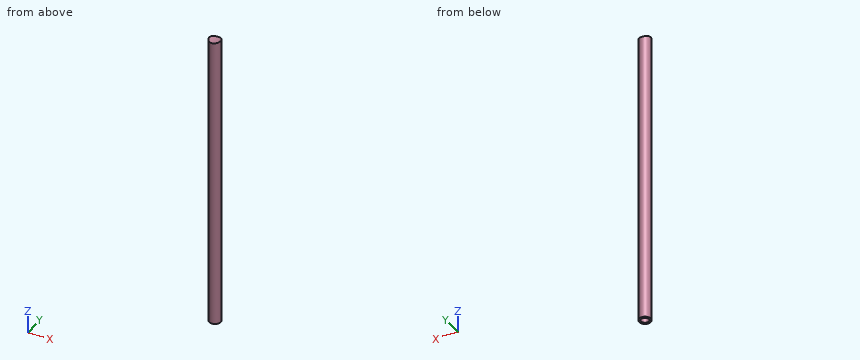
Autodesk Inventor part; units mm, degrees
ref_plane "Start Plane" through (0, 0, 0) normal (0, 0, 1) x (1, 0, 0)
ref_plane "End Plane" through (0, 0, 340) normal (0, 0, 1) x (1, 0, 0)
ref_plane "YZ Plane" through (0, 0, 0) normal (1, 0, 0) x (0, 1, 0)
ref_plane "Start Plane" through (0, 0, 0) normal (0, 0, 1) x (1, 0, 0)
ref_plane "End Plane" through (0, 0, 340) normal (0, 0, 1) x (1, 0, 0)
sketch "Sketch" plane through (0, 0, 0) normal (0, 0, 1) x (1, 0, 0)
  circle A0 centre (0, 0) radius 6.35
  dimension "d0" = 12.7
extrude "Body" add sketch "Sketch" along normal up to surface (340 mm away) from surface at 0
sketch "Sketch2" plane through (0, 0, 0) normal (0, 0, 1) x (1, 0, 0)
  line L0 (0, 0) -> (10, 0)
ref_plane "Work Plane3" through (0, 0, 0) normal (0, -1, 0) x (1, 0, 0)
sketch "Sketch4" plane through (0, 0, 0) normal (0, 1, 0) x (-1, 0, 0)
  line L0 (-6.35, 340) -> (6.35, 340)
  circle A0 centre (0, 340) radius 20
  point P0 (0, 0)
  dimension "d11" = 40
extrude "Extrusion2" cut sketch "Sketch4" along normal through all both and the other way through all
sketch "Sketch5" plane through (0, 0, 0) normal (0, 0, -1) x (-1, 0, 0)
  circle A0 centre (0, 0) radius 4.2164
  dimension "d12" = 8.4328
extrude "Extrusion3" cut sketch "Sketch5" against normal blind 50.8
thread "Thread1"
sketch "Sketch3" plane through (0, 0, 0) normal (0, -1, 0) x (1, 0, 0)
  line L0 (-2, 0) -> (12, 0)
  line L1 (-2, 340) -> (12, 340)
  dimension "d7" = 340
equation "\"d0\" = Diam"
equation "\"d1\" = G_L"
equation "\"Diam\" = 12.7"
equation "\"G_L\" = d7"
equation "\"G_OFFSET_START\" = 0"
equation "\"G_OFFSET_END\" = 0"
equation "\"d5\" = G_OFFSET_END + B_L"
equation "\"B_L\" = 340"
properties part number "ANSI/AISC Rolled Steel - 1/2-13.386, RB" material "Steel, Mild"
Verification items for the finished model (mm, model axes). Coordinates: 2 decimals unless noted, no trailing zeros. Write each loop counter-clockwise with the first axis right and the second up, starting at its lowest first coordinate (ties: lowest second). Pieces come first, ordered by that corner, then holes. Notation, with made-up numbers: (-37, 45) - (-26, 45) arc R8 ccw to (-26, 59) - close; hole circle Ø11 at (68.25, 27.5). An arc over 180 degrees is marked (long way). One line per question, with ' | ' between items. Start each with the question number.
1. Section check B-B (x = 0). Enter the section's corners in (y, z), plus the area to 3 significant figures.
2. Gauge pin test, flat ends, axial feed: P1, Ø1, axis at x = -0.5, y = -4.5, coming from the +Z side (3 decimals); P2, Ø3, axis at x = 3.5, z = 254, coming from the +Y side; P3, Ø4, axis at x = 0, y = -5, coming from the -Z side; P4, Ø1.5, axis at x = -3.5, z = 244, coming from the -Y side. Record the tip position at first contact, or that the pin passes through.
3. Material ranges on line 1 along Y through (x, z) = (0, 20.5); line 2 along Z through (x, y) = (-0.25, 3.5); line 3 along X through (y, z) = (-0.25, 288), recorded low to high.
4. Section check C-C (z = 88). Enter the section's corners in (x, y).
5. Section check A-A (y = 0). Enter the section's corners in (x, z).
Computed values:
1) outline: (-6.35, 0) - (-4.22, 0) - (-4.22, 50.8) - (4.22, 50.8) - (4.22, 0) - (6.35, 0) - (6.35, 320) - (-6.35, 320) - close | area: 3,640 mm²
2) P1: z = 320.025 | P2: y = 6.03 | P3: z = 0 | P4: y = -5.72
3) line 1: -6.35 to -4.22, 4.22 to 6.35 | line 2: 50.8 to 320 | line 3: -6.35 to 6.35
4) outline: circle Ø12.7 at (0, 0)
5) outline: (-6.35, 0) - (-4.22, 0) - (-4.22, 50.8) - (4.22, 50.8) - (4.22, 0) - (6.35, 0) - (6.35, 321.03) arc R20 cw to (-6.35, 321.03) - close
